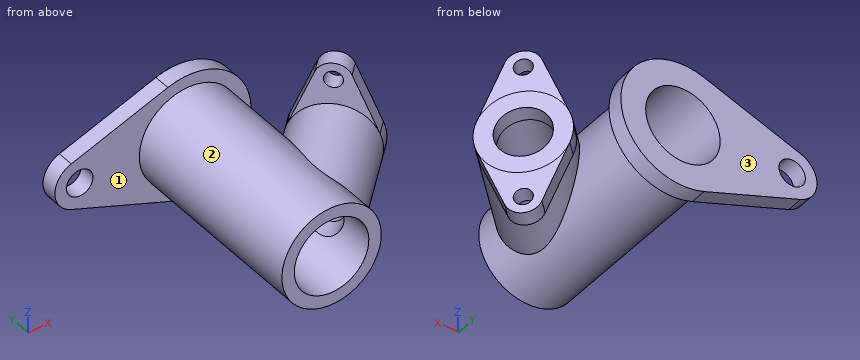
```python
from build123d import *
from build123d.topology import SkipClean

# Parameters (mm, degrees)
SKETCH_1_R                      = 60
EXTRUDE_1_DEPTH                 = 240
SKETCH_2_R                      = 16
EXTRUDE_2_DEPTH                 = 20
CUT_EXTRUDE_1_DEPTH             = 316.38706378
CUT_EXTRUDE_1_DEPTH_BACK        = 316.38706378
SKETCH_6_R                      = 45
EXTRUDE_3_REACH                 = 335.721
EXTRUDE_3_END_RADIUS            = 60
SKETCH_5_R                      = 50
SKETCH_5_R_2                    = 30
CUT_EXTRUDE_2_REACH             = 343.929
SKETCH_8_R                      = 30
CUT_EXTRUDE_2_DIRECTION_2_DEPTH = 342.928852652
SKETCH_9_R                      = 10
SKETCH_9_R_2                    = 30
EXTRUDE_4_DEPTH                 = 20


with BuildPart() as part:
    # 草图1 → 凸台-拉伸1 (new body)
    with BuildSketch(Plane(origin=(0, 0, 0), x_dir=(1, 0, 0), z_dir=(0, 1, 0))):
        with Locations(Location((0, 0, 0), (0, 0, 270))):
            Circle(SKETCH_1_R)
    extrude(amount=EXTRUDE_1_DEPTH)

    # 草图2 → 凸台-拉伸2 (add)
    with BuildSketch(Plane(origin=(0, 240, 0), x_dir=(1, 0, 0), z_dir=(0, 1, 0))):
        with BuildLine():
            Line((-142.227272727, 28.202888018), (-25.568181818, 70.507220045))
            ThreePointArc((-25.568181818, 70.507220045), (75, 0), (-25.568181818, -70.507220045))
            Line((-25.568181818, -70.507220045), (-142.227272727, -28.202888018))
            ThreePointArc((-142.227272727, -28.202888018), (-162, 0), (-142.227272727, 28.202888018))
        make_face()
        with Locations(Location((-132, 0, 0), (0, 0, 270))):
            Circle(SKETCH_2_R, mode=Mode.SUBTRACT)
    extrude(amount=EXTRUDE_2_DEPTH)

    # 草图6 → 切除-拉伸1 (cut, two sides: drawn at the far end of the back side and taken through both)
    with BuildSketch(Plane(origin=(0, 260, 0), x_dir=(1, 0, 0), z_dir=(0, 1, 0)).offset(-CUT_EXTRUDE_1_DEPTH_BACK)):
        with Locations(Location((0, 0, 0), (0, 0, 270))):
            Circle(SKETCH_6_R)
    extrude(amount=CUT_EXTRUDE_1_DEPTH + CUT_EXTRUDE_1_DEPTH_BACK, mode=Mode.SUBTRACT)

    # 凸台-拉伸3: up to this cylinder (the profile starts outside it)
    extrude_3_end = Plane(origin=(0, 125.644661, 0), z_dir=(0, -1, 0)) * Cylinder(EXTRUDE_3_END_RADIUS, 792.442, mode=Mode.PRIVATE)
    # 草图5 → 凸台-拉伸3 (add, up to the surface)
    with BuildSketch(Plane(origin=(121.098951134, 160, 0), x_dir=(0.7071067811865488, -0.7071067811865464, 0), z_dir=(0.7071067811865464, 0.7071067811865488, 0)), mode=Mode.PRIVATE) as extrude_3_sk1:
        with Locations(Location((0, 0, 0), (0, 0, 180))):
            Circle(SKETCH_5_R)
        with Locations(Location((0, 0, 0), (0, 0, 180))):
            Circle(SKETCH_5_R_2, mode=Mode.SUBTRACT)
    extrude_3_tool1 = extrude(extrude_3_sk1.sketch, amount=-EXTRUDE_3_REACH, mode=Mode.PRIVATE) - extrude_3_end
    add(extrude_3_tool1.solids().sort_by_distance((155.45429, 125.644661, 0))[0])

    # 草图8 → 切除-拉伸2 (cut, up to next)
    with BuildSketch(Plane(origin=(140.549475567, 140.549475567, 0), x_dir=(0, 0, -1), z_dir=(0.7071067811865465, 0.7071067811865487, 0)), mode=Mode.PRIVATE) as cut_extrude_2_sk1:
        with Locations(Location((0, 27.507195448, 0), (0, 0, 90))):
            Circle(SKETCH_8_R)
    cut_extrude_2_tool1 = extrude(cut_extrude_2_sk1.sketch, amount=-CUT_EXTRUDE_2_REACH, mode=Mode.PRIVATE) & part.part
    add(cut_extrude_2_tool1.solids().sort_by_distance((121.098951, 160, 0))[0], mode=Mode.SUBTRACT)

    # 草图8 → 切除-拉伸2 direction 2 (cut)
    with BuildSketch(Plane(origin=(140.549475567, 140.549475567, 0), x_dir=(0, 0, -1), z_dir=(0.7071067811865465, 0.7071067811865487, 0))):
        with Locations(Location((0, 27.507195448, 0), (0, 0, 90))):
            Circle(SKETCH_8_R)
    extrude(amount=CUT_EXTRUDE_2_DIRECTION_2_DEPTH, mode=Mode.SUBTRACT)

    # 草图9 → 凸台-拉伸4 (add)
    with SkipClean():  # the faces are left unmerged after this step: merging them gives an invalid solid
        with BuildSketch(Plane(origin=(140.549475567, 140.549475567, 0), x_dir=(0, 0, -1), z_dir=(0.7071067811865465, 0.7071067811865487, 0))):
            with BuildLine():
                Line((-87.5, 46.047691666), (-18.75, 73.858435993))
                ThreePointArc((-18.75, 73.858435993), (0, 77.507195448), (18.75, 73.858435993))
                Line((18.75, 73.858435993), (87.5, 46.047691666))
                ThreePointArc((87.5, 46.047691666), (100, 27.507195448), (87.5, 8.966699231))
                Line((87.5, 8.966699231), (18.75, -18.844045096))
                ThreePointArc((18.75, -18.844045096), (0, -22.492804552), (-18.75, -18.844045096))
                Line((-18.75, -18.844045096), (-87.5, 8.966699231))
                ThreePointArc((-87.5, 8.966699231), (-100, 27.507195448), (-87.5, 46.047691666))
            make_face()
            with Locations(Location((-80, 27.507195448, 0), (0, 0, 90))):
                Circle(SKETCH_9_R, mode=Mode.SUBTRACT)
            with Locations(Location((80, 27.507195448, 0), (0, 0, 90))):
                Circle(SKETCH_9_R, mode=Mode.SUBTRACT)
            with Locations(Location((0, 27.507195448, 0), (0, 0, 90))):
                Circle(SKETCH_9_R_2, mode=Mode.SUBTRACT)
        extrude(amount=-EXTRUDE_4_DEPTH)


solid = part.part
```
Geometry check sheet. Reference: the model listing, model coordinates, mm. Face numbers are marked on the shaded views. Coordinates: 2 decimals unless noted, no trailing zeros. Write each loop counter-clockwise with the first axis right and the second up, starting at its lowest first coordinate (ties: lowest second). Pieces come first, ordered by that corner, then holes. Notation, with made-up numbers: M -29,-30.5 L 17,-30.5 A21 cw 17,3.5 Z; hole C 13.5,-10.75 d2. An arc over 180 degrees is marked long. One line per item, written item: value. Start each with the question number.
(1) Release check for a two-part mould opening along Y. For the marked faces 1, 2 and 3 record: released by +Y, released by -Y, zero draft, split by the parting line, or undercut.
(2) Scan lines: line 1 along X through (y, z) = (187, 16); line 2 along Y through (x, z) = (-100, -41); line 3 along X through (y, z) = (186, 0). Record each from-to range of solid material in increasing order. Write a range as [from, to].
(3) Sectioned sample at A-A, the plane x = 0. Enter the section's corners in (y, z), and give its area (3 significant figures).
(4) Sectioned sample at D-D, the plane x = -132. Enter the section's corners in (y, z), and give its area (3 significant figures).
(5) Sectioned sample at C-C, the plane y = 211.5. Enter the section's corners in (x, z), and give its area (3 significant figures).
(6) Depth check by flat-ended pin: pin 1 (2 mm diameter, centred on x = -92.5, z = 38, fed in from -Y); pin 2 (1.5 mm diameter, centred on x = 31, y = 152, fed in from +Z); pin 3 (3 mm diameter, centred on y = 180, z = 30.5, fed in from +X). Enter the tip coordinate at first touch or a pass-through.
Filled sheet:
1. face 1: undercut
1. face 2: undercut
1. face 3: released by +Y
2. line 1: [-57.83, -42.06], [42.06, 57.83], [81.11, 94.1]
2. line 2: [240, 260]
2. line 3: [-60, -45], [45, 60], [76.39, 95.1]
3. outline: M 0,-60 L 240,-60 L 240,-75 L 260,-75 L 260,-45 L 0,-45 Z; M 0,45 L 260,45 L 260,75 L 240,75 L 240,60 L 0,60 Z
3. area: 8,400 mm²
4. outline: M 240,-31.91 L 260,-31.91 L 260,-16 L 240,-16 Z; M 240,16 L 260,16 L 260,31.91 L 240,31.91 Z
4. area: 636 mm²
5. outline: C 0,0 d120; hole C 0,0 d90
5. area: 4,950 mm²
6. pin 1: y = 240
6. pin 2: z = 51.82
6. pin 3: x = 102.6
